from build123d import *

# Parameters (mm, degrees)
SKETCH_1_R          = 3.5
EXTRUDE_1_DEPTH     = 12
SKETCH_2_R          = 2.125
CUT_EXTRUDE_1_DEPTH = 12
SKETCH_3_R          = 1.5
CUT_EXTRUDE_2_DEPTH = 12
CUT_EXTRUDE_3_DEPTH = 5


with BuildPart() as part:
    # 草图1 → 凸台-拉伸1 (new body)
    with BuildSketch(Plane(origin=(0, 0, 0), x_dir=(1, 0, 0), z_dir=(0, 1, 0))):
        with Locations(Location((0, 0, 0), (0, 0, 270))):
            Circle(SKETCH_1_R)
    extrude(amount=EXTRUDE_1_DEPTH)

    # 草图2 → 切除-拉伸1 (cut)
    with BuildSketch(Plane(origin=(0, 12, 0), x_dir=(1, 0, 0), z_dir=(0, 1, 0))):
        with Locations(Location((0, 0, 0), (0, 0, 270))):
            Circle(SKETCH_2_R)
    extrude(amount=-CUT_EXTRUDE_1_DEPTH, mode=Mode.SUBTRACT)

    # 草图3 → 切除-拉伸2 (cut)
    with BuildSketch(Plane(origin=(0, 0, 0), x_dir=(0, 0, -1), z_dir=(1, 0, 0))):
        with Locations((0, 2.692201217)):
            Circle(SKETCH_3_R)
    extrude(amount=-CUT_EXTRUDE_2_DEPTH, mode=Mode.SUBTRACT)

    # 草图4 → 切除-拉伸3 (cut)
    with BuildSketch(Plane(origin=(0, 12, 0), x_dir=(1, 0, 0), z_dir=(0, 1, 0))):
        with BuildLine():
            Line((-1.975, 1.913602623), (-1.975, -1.913602623))
            ThreePointArc((-1.975, -1.913602623), (0, -2.75), (1.975, -1.913602623))
            Line((1.975, -1.913602623), (1.975, 1.913602623))
            ThreePointArc((1.975, 1.913602623), (0, 2.75), (-1.975, 1.913602623))
        make_face()
    extrude(amount=-CUT_EXTRUDE_3_DEPTH, mode=Mode.SUBTRACT)


solid = part.part
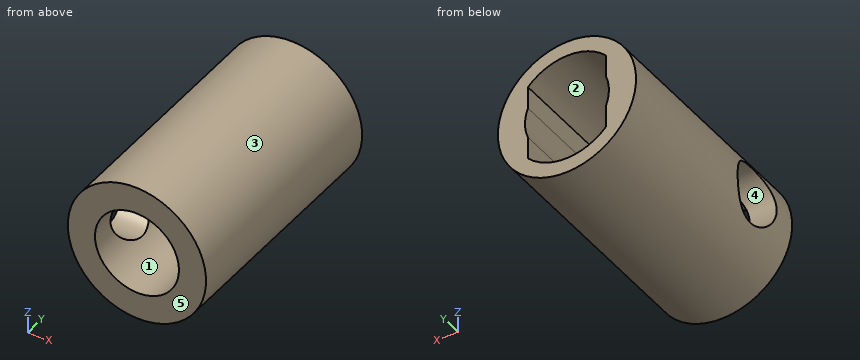
Read the model definition and answer for the solid it produces. Units are mm, in the model's axes. Face numbers are marked on the shaded views. A direction names the side the tool comes from. Coordinates: 2 decimals unless noted, no trailing zeros. Order: outer loops, then holes, each group sorted by start corner. A loop starts at its lowest first (then second) coordinate and runs counter-clockwise, first axis right, second up. Notation, with made-up numbers: (0.25, 62.25) -> (12.25, 62.25) arc R22 ccw to (12.25, 81.25) -> close; hole circle Ø2 at (-33, 87.5). An arc over 180 degrees is marked (long way). Answer as a JSON object with one key per item and string values.
1) A cutting plane is placed at B-B, the plane z = 0. Determine the outline of the cut face in (x, y) (3 decimals), plus the area to 3 significant figures.
Model answer:
{"outline": "(-3.5, 0) -> (-2.125, 0) -> (-2.125, 1.192) -> (-3.5, 1.192) -> close; (-3.5, 4.192) -> (-2.125, 4.192) -> (-2.125, 12) -> (-3.5, 12) -> close; (2.125, 0) -> (3.5, 0) -> (3.5, 12) -> (2.125, 12) -> close", "area": "28.9 mm²"}
2) A cutting plane is placed at D-D, the plane z = -1.75. Determine the outline of the cut face in (x, y) (3 decimals).
Model answer:
{"outline": "(-3.031, 0) -> (-1.205, 0) -> (-1.205, 7) -> (-1.975, 7) -> (-1.975, 12) -> (-3.031, 12) -> close; (1.205, 0) -> (3.031, 0) -> (3.031, 12) -> (1.975, 12) -> (1.975, 7) -> (1.205, 7) -> close"}
3) The mould has two halves that part along Z. Classify the marked faces 3, 4 and 5: released by +Z, released by -Z, zero draft, split by the parting line, or undercut.
Model answer:
{"face 3": "split by the parting line", "face 4": "undercut", "face 5": "zero draft"}
4) Each of these flat-tipped pins is pushed along its axis until it touches: pin 1 (1.5 mm diameter, centred on y = 3.5, z = -1, fed in from -X); pin 2 (0.9 mm diameter, centred on y = 10.5, z = -1, fed in from +X); pin 3 (2.5 mm diameter, centred on x = 0, z = 0, fed in from +Y); pin 4 (1.5 mm diameter, centred on x = -1, y = 6, fed in from -Z). Where does it stop, or does it pass through?
Model answer:
{"pin 1": "stops at x = -3.46", "pin 2": "stops at x = 3.46", "pin 3": "passes through", "pin 4": "stops at z = -3.49"}
5) A tool of negligible diameter and unlimited length cuts with its end or side. For the marked faces 1 and 2, from which of +Z, -Z, +X, -X, +Y, -Y can it reach the whole face along a straight path? Write none if from no direction.
Model answer:
{"face 1": "+Y, -Y", "face 2": "+Y"}
6) Consider line 1 along X through (y, z) = (0.5, 0) (3 decimals); line 2 along Y through (x, z) = (-2.7, 0); line 3 along Y through (x, z) = (-1, 2). Determine where each line is inside the solid, lowest interval first. Write a range as from..to.
Model answer:
{"line 1": "x = -3.5..-2.125, 2.125..3.5", "line 2": "y = 0..1.19, 4.19..12", "line 3": "y = 0..7"}
7) A cutting plane is placed at C-C, the plane y = 10. Determine the outline of the cut face in (x, z) (3 decimals), plus the area to 3 significant figures.
Model answer:
{"outline": "circle Ø7 at (0, 0); hole (-1.975, -1.914) arc R2.75 ccw to (1.975, -1.914) -> (1.975, -0.784) arc R2.125 ccw to (1.975, 0.784) -> (1.975, 1.914) arc R2.75 ccw to (-1.975, 1.914) -> (-1.975, 0.784) arc R2.125 ccw to (-1.975, -0.784) -> close", "area": "18.5 mm²"}
8) A cutting plane is placed at A-A, the plane x = 0. Determine the outline of the cut face in (y, z) (3 decimals).
Model answer:
{"outline": "(0, -3.5) -> (12, -3.5) -> (12, -2.75) -> (7, -2.75) -> (7, -2.125) -> (0, -2.125) -> close; (0, 2.125) -> (7, 2.125) -> (7, 2.75) -> (12, 2.75) -> (12, 3.5) -> (0, 3.5) -> close"}
